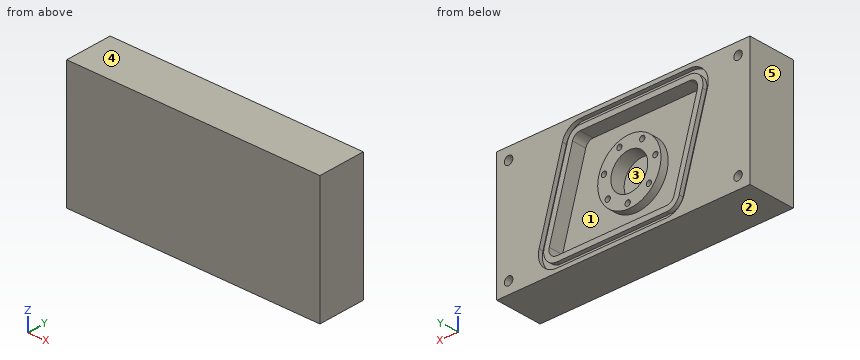
```python
from build123d import *

# Parameters (mm, degrees)
SKETCH1_W                      = 152.4
SKETCH1_H                      = 76.2
BOSS_EXTRUDE1_DEPTH            = 28.575
F_7_0_201_DIAMETER_HOLE1_D     = 5.1054
F_7_0_201_DIAMETER_HOLE1_DEPTH = 12.7
F_7_0_201_DIAMETER_HOLE1_TIP   = 1.533816902
SKETCH4_R                      = 11.1125
CUT_EXTRUDE1_DEPTH             = 12.7
CIRPATTERN2_COUNT              = 7
SKETCH9_R                      = 19.05
CUT_EXTRUDE5_DEPTH             = 3.9624
SKETCH10_R                     = 19.05
CUT_EXTRUDE6_DEPTH             = 8.7122
CUT_EXTRUDE7_DEPTH             = 2.5908


with BuildPart() as part:
    # Sketch1 → Boss-Extrude1 (new body)
    with BuildSketch(Plane(origin=(0, 0, 0), x_dir=(1, 0, 0), z_dir=(0, 1, 0))):
        Rectangle(SKETCH1_W, SKETCH1_H)
    extrude(amount=BOSS_EXTRUDE1_DEPTH)

    # #7 (0.201) Diameter Hole1
    with Locations(Plane(origin=(0, 28.575, 0), x_dir=(-1, 0, 0), z_dir=(0, 1, 0))):
        with Locations((69.0626, -30.9626), (69.0626, 30.9626), (-69.0626, 30.9626), (-69.0626, -30.9626)):
            Hole(F_7_0_201_DIAMETER_HOLE1_D / 2, depth=F_7_0_201_DIAMETER_HOLE1_DEPTH)
            with Locations((0, 0, -(F_7_0_201_DIAMETER_HOLE1_DEPTH + F_7_0_201_DIAMETER_HOLE1_TIP / 2))):  # 118° drill point
                Cone(0, F_7_0_201_DIAMETER_HOLE1_D / 2, F_7_0_201_DIAMETER_HOLE1_TIP, mode=Mode.SUBTRACT)

    # Sketch4 → Cut-Extrude1 (cut)
    with BuildSketch(Plane(origin=(0, 28.575, 0), x_dir=(1, 0, 0), z_dir=(0, 1, 0))):
        Circle(SKETCH4_R)
    extrude(amount=-CUT_EXTRUDE1_DEPTH, mode=Mode.SUBTRACT)

    # Sketch14 → 1/8 (0.125) Diameter Hole2 (revolve, cut)
    with BuildSketch(Plane(origin=(13.004038703, 28.575, -9.105525927), x_dir=(0, 0, 1), z_dir=(1, 0, 0))):
        Polygon((0, 0), (0, 13.653866233), (1.5875, 12.7), (1.5875, 0), align=None)
    f_1_8_0_125_diameter_hole2 = revolve(axis=Axis((13.004038703, 34.925, -9.105525927), (0, -1, 0)), mode=Mode.SUBTRACT)

    # CirPattern2: 1/8 (0.125) Diameter Hole2 ×7 about axis
    cirpattern2_axis = Axis((0, 0, 0), (0, 1, 0))
    for i in range(1, CIRPATTERN2_COUNT):
        add(f_1_8_0_125_diameter_hole2.rotate(cirpattern2_axis, i * 360 / CIRPATTERN2_COUNT), mode=Mode.SUBTRACT)

    # Sketch9 → Cut-Extrude5 (cut)
    with BuildSketch(Plane(origin=(0, 28.575, 0), x_dir=(1, 0, 0), z_dir=(0, 1, 0))):
        Circle(SKETCH9_R)
    extrude(amount=-CUT_EXTRUDE5_DEPTH, mode=Mode.SUBTRACT)

    # Sketch10 → Cut-Extrude6 (cut)
    with BuildSketch(Plane(origin=(0, 28.575, 0), x_dir=(1, 0, 0), z_dir=(0, 1, 0))):
        with BuildLine():
            Line((-25.9842, 29.3624), (40.005, 29.3624))
            ThreePointArc((40.005, 29.3624), (43.806157259, 27.469152471), (44.585149022, 23.294663934))
            Line((44.585149022, 23.294663934), (30.564349022, -25.905136066))
            ThreePointArc((30.564349022, -25.905136066), (28.853452471, -28.401057259), (25.9842, -29.3624))
            Line((25.9842, -29.3624), (-40.005, -29.3624))
            ThreePointArc((-40.005, -29.3624), (-43.806157259, -27.469152471), (-44.585149022, -23.294663934))
            Line((-44.585149022, -23.294663934), (-30.564349022, 25.905136066))
            ThreePointArc((-30.564349022, 25.905136066), (-28.853452471, 28.401057259), (-25.9842, 29.3624))
        make_face()
        Circle(SKETCH10_R, mode=Mode.SUBTRACT)
    extrude(amount=-CUT_EXTRUDE6_DEPTH, mode=Mode.SUBTRACT)

    # Sketch11 → Cut-Extrude7 (cut)
    with BuildSketch(Plane(origin=(0, 28.575, 0), x_dir=(1, 0, 0), z_dir=(0, 1, 0))):
        with BuildLine():
            Line((-36.671214384, 27.645450821), (-50.692014384, -21.554349179))
            ThreePointArc((-50.692014384, -21.554349179), (-48.874366938, -31.294822432), (-40.005, -35.7124))
            Line((-40.005, -35.7124), (25.9842, -35.7124))
            ThreePointArc((25.9842, -35.7124), (32.679122432, -33.469266938), (36.671214384, -27.645450821))
            Line((36.671214384, -27.645450821), (50.692014384, 21.554349179))
            ThreePointArc((50.692014384, 21.554349179), (48.874366938, 31.294822432), (40.005, 35.7124))
            Line((40.005, 35.7124), (-25.9842, 35.7124))
            ThreePointArc((-25.9842, 35.7124), (-32.679122432, 33.469266938), (-36.671214384, 27.645450821))
        make_face()
        with BuildLine():
            Line((-33.617781703, 26.775293443), (-47.638581703, -22.424506557))
            ThreePointArc((-47.638581703, -22.424506557), (-46.340262098, -29.381987452), (-40.005, -32.5374))
            Line((-40.005, -32.5374), (25.9842, -32.5374))
            ThreePointArc((25.9842, -32.5374), (30.766287452, -30.935162098), (33.617781703, -26.775293443))
            Line((33.617781703, -26.775293443), (47.638581703, 22.424506557))
            ThreePointArc((47.638581703, 22.424506557), (46.340262098, 29.381987452), (40.005, 32.5374))
            Line((40.005, 32.5374), (-25.9842, 32.5374))
            ThreePointArc((-25.9842, 32.5374), (-30.766287452, 30.935162098), (-33.617781703, 26.775293443))
        make_face(mode=Mode.SUBTRACT)
    extrude(amount=-CUT_EXTRUDE7_DEPTH, mode=Mode.SUBTRACT)


solid = part.part
```
Build history of the part. All positions in model axes, mm. Face numbers are marked on the shaded views. A direction names the side the tool comes from. Coordinates: 2 decimals unless noted, no trailing zeros. Order: outer loops, then holes, each group sorted by start corner. A loop starts at its lowest first (then second) coordinate and runs counter-clockwise, first axis right, second up.
Item 1: Mould opens along X. For the marked faces 3, 4 and 5 say: released by +X, released by -X, zero draft, split by the parting line, or undercut.
Filled in:
face 3: undercut
face 4: zero draft
face 5: released by -X
Item 2: Drop flat-ended pins along their axis: pin 1 Ø21.5 at (x, z) = (17, -11.5) entering from +Y; pin 2 Ø2.5 at (x, z) = (15.23, 4.49) entering from +Y; pin 3 Ø2.5 at (x, z) = (-15.67, 2.56) entering from -Y; pin 4 Ø5 at (x, z) = (0, -1) entering from +Y (3 decimals). Give the stop position or say it passes through.
Filled in:
pin 1: stops at y = 24.61
pin 2: stops at y = 15.67
pin 3: stops at y = 0
pin 4: stops at y = 15.875
Item 3: Tool access for the marked faces 1 and 2: list every direction of +Z, -Z, +X, -X, +Y, -Y with a clear straight run to the whole face (end or side of a thin tool).
Filled in:
face 1: +Y
face 2: -Z, +X, -X, +Y, -Y
Item 4: Drill centre lines: L1, parallel to Z at x = 0, y = 22.5; L2, parallel to Z at x = 16, y = 20.5; L3, parallel to Y at x = -18, z = -14. Where is each one in solid material? Low to high.
Filled in:
L1: z = -38.1 to -29.36, -19.05 to -17.09, -14.6 to -11.11, 11.11 to 19.05, 29.36 to 38.1
L2: z = -38.1 to -29.36, -10.34 to 3.1, 5.88 to 10.34, 29.36 to 38.1
L3: y = 0 to 19.86
Item 5: Saw through at A-A on x = -24.5. List the corners of the cut face in (y, z) (3 decimals), then the cut area to 3 significant figures.
Filled in:
outline: (0, -38.1) - (28.575, -38.1) - (28.575, -35.712) - (25.984, -35.712) - (25.984, -32.537) - (28.575, -32.537) - (28.575, -29.362) - (19.863, -29.362) - (19.863, 29.362) - (28.575, 29.362) - (28.575, 32.537) - (25.984, 32.537) - (25.984, 35.712) - (28.575, 35.712) - (28.575, 38.1) - (0, 38.1) - close
area: 1,650 mm2
